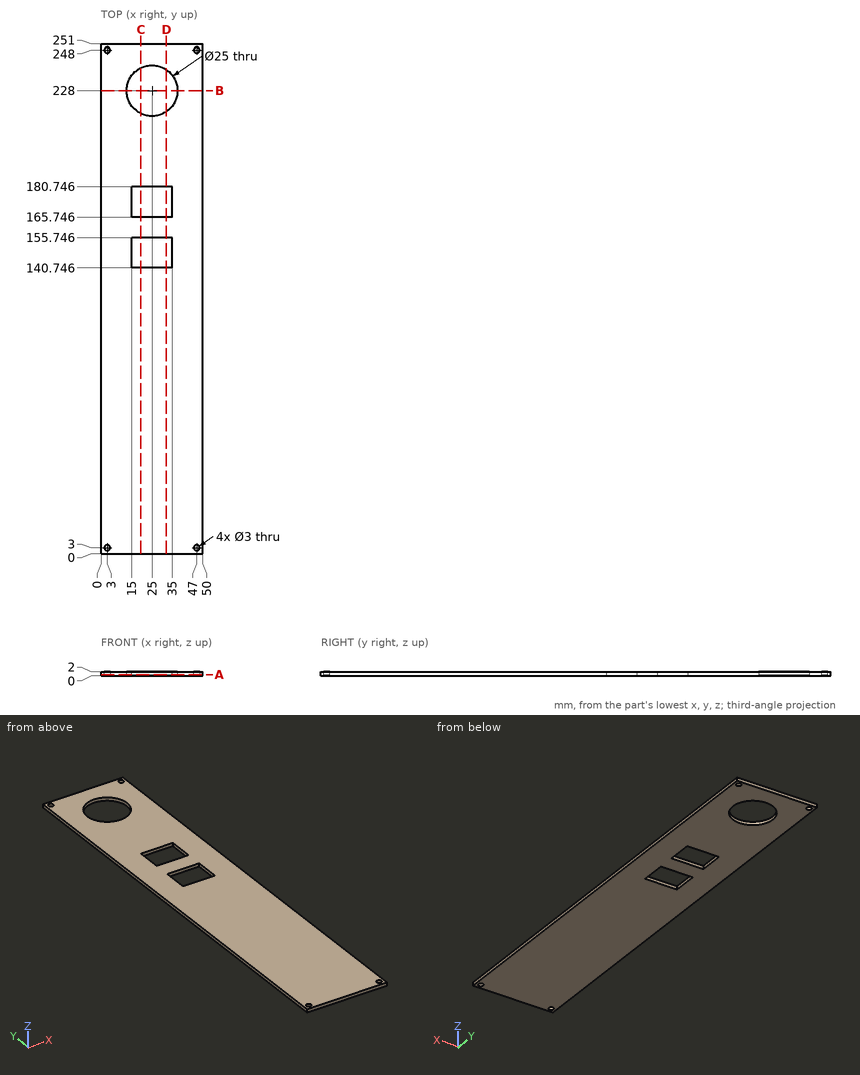
Answer from the drawing. Dimensions are ordinates in mm from the lowest x, y and z of the part. Coordinates: 2 decimals unless noted, no trailing zeros. Loops run counter-clockwise (first coordinate to the right, second up) from the corner with the lowest first, then second, coordinate; pieces in that order, holes last.
1) Section D-D (x = 32) is taken. Give the vertices of the cut face in (y, z).
Results:
outline: (0, 0) - (140.75, 0) - (140.75, 2) - (0, 2) - close; (155.75, 0) - (165.75, 0) - (165.75, 2) - (155.75, 2) - close; (180.75, 0) - (217.64, 0) - (217.64, 2) - (180.75, 2) - close; (238.36, 0) - (251, 0) - (251, 2) - (238.36, 2) - close
2) Section A-A (z = 0.7) is taken. Give the vertices of the cut face in (x, y), plus the area to 3 significant figures.
Results:
outline: (0, 0) - (50, 0) - (50, 251) - (0, 251) - close; hole circle Ø3 at (3, 3); hole circle Ø3 at (3, 248); hole circle Ø25 at (25, 228); hole (15, 140.75) - (35, 140.75) - (35, 155.75) - (15, 155.75) - close; hole (15, 165.75) - (35, 165.75) - (35, 180.75) - (15, 180.75) - close; hole circle Ø3 at (47, 3); hole circle Ø3 at (47, 248)
area: 11,400 mm2
3) Section B-B (y = 228) is taken. Give the vertices of the cut face in (x, z), plus the area to 3 significant figures.
Results:
outline: (0, 0) - (12.5, 0) - (12.5, 2) - (0, 2) - close; (37.5, 0) - (50, 0) - (50, 2) - (37.5, 2) - close
area: 50.0 mm2
4) Flat-ended cylindrical pins translate along their axes: pin 1 (3.5 mm diameter, centred on x = 47, y = 3, fed in from +Z); pin 2 (2.5 mm diameter, centred on x = 3, y = 3, fed in from +Z). Find the tip coordinate at first contact, or state that the pin passes through.
Results:
pin 1: stops at z = 2
pin 2: passes through
5) Section C-C (x = 19.5) is taken. Give the vertices of the cut face in (y, z) (1 decimal).
Results:
outline: (0, 0) - (140.7, 0) - (140.7, 2) - (0, 2) - close; (155.7, 0) - (165.7, 0) - (165.7, 2) - (155.7, 2) - close; (180.7, 0) - (216.8, 0) - (216.8, 2) - (180.7, 2) - close; (239.2, 0) - (251, 0) - (251, 2) - (239.2, 2) - close
6) Consider probe 1 along X at (y, z) = (3, 0.8); probe 2 along Y at (x, z) = (47, 0.45); probe 3 along X at (y, z) = (178, 0.95). Determine where each line is inside the solid, lowest interval first.
Results:
probe 1: x = 0 to 1.5, 4.5 to 45.5, 48.5 to 50
probe 2: y = 0 to 1.5, 4.5 to 246.5, 249.5 to 251
probe 3: x = 0 to 15, 35 to 50
